from build123d import *

# Parameters (mm, degrees)
F0_W     = 10
F0_H     = 40
F0_H_2   = 20
F1_DEPTH = 120
F2_DEPTH = 30
F3_DEPTH = 100


with BuildPart() as f1:
    # F0 (on Top) → F1 (new body)
    with BuildSketch(Plane.XY):
        with Locations((5, 40)):
            Rectangle(F0_W, F0_H)
        Polygon((10, 20), (30, 20), (40, 20), (40, 40), (20, 40), (20, 60), (10, 60), align=None)
        with Locations((35, 10)):
            Rectangle(F0_W, F0_H_2)
        Polygon((0, 20), (0, 0), (30, 0), (30, 20), (10, 20), align=None)
    extrude(amount=-F1_DEPTH)

    # F0 (on Top) → F2 (cut)
    with BuildSketch(Plane.XY):
        with Locations((35, 10)):
            Rectangle(F0_W, F0_H_2)
        Polygon((10, 20), (30, 20), (40, 20), (40, 40), (20, 40), (20, 60), (10, 60), align=None)
    extrude(amount=-F2_DEPTH, mode=Mode.SUBTRACT)

    # F0 (on Top) → F3 (cut)
    with BuildSketch(Plane.XY):
        Polygon((10, 20), (30, 20), (40, 20), (40, 40), (20, 40), (20, 60), (10, 60), align=None)
    extrude(amount=-F3_DEPTH, mode=Mode.SUBTRACT)


solid = f1.part
Source: CAD feature listing. Evaluate the final solid. Frame: model axes, mm. A direction names the side the tool comes from. Give positions to 0.01 mm unless a question says otherwise; leave off trailing zeros. Write each loop counter-clockwise with the first axis right and the second up, starting at its lowest first coordinate (ties: lowest second). Pieces come first, ordered by that corner, then holes. Notation, with made-up numbers: M 75.5,7.5 L 115.5,7.5 A25 cw 115.5,29.5 Z; hole C -29.75,-27.75 d10. An arc over 180 degrees is marked long. Return JSON: item names as keys, results as strings. Group by question number.
1) Pin query (flat end, axial travel): P1, Ø10, axis at y = 53.5, z = -54.5, coming from the -X side; P2, Ø4, axis at y = 53, z = -43, coming from the +X side; P3, Ø10, axis at y = 51.5, z = -110, coming from the +X side; P4, Ø10, axis at x = 33.5, z = -110, coming from the +Y side. Return the tip coordinate at first contact, or that it passes through.
2) Cut plane A-A, the plane y = 38. Output: boundary loops of the cut face in (x, z).
3) Set-up query: faces 1 (the face through (30, 10, -15)), 2 (the face through (30, 40, -110)), 3 (the face through (21, 36, -100)). Return all of +Z, -Z, +X, -X, +Y, -Y with unobstructed straight access to the full face (end or side cutting, diameter ignored); none if empty.
4) Material intervals for line 1 along Y through (x, z) = (13, -62); line 2 along X through (y, z) = (43, -26); line 3 along Z through (x, y) = (19.5, 26), sorted ascending. Write a range as [from, to].
5) Cut plane B-B, the plane x = 12. Output: boundary loops of the cut face in (y, z), plus the area to 3 significant figures.
Recorded:
{
 "1": {"P1": "stops at x = 0", "P2": "stops at x = 10", "P3": "stops at x = 20", "P4": "stops at y = 40"},
 "2": {"outline": "M 0,-120 L 40,-120 L 40,-100 L 10,-100 L 10,0 L 0,0 Z"},
 "3": {"face 1": "+Z, +X, +Y, -Y", "face 2": "+Z, -Z, +X, +Y", "face 3": "+Z, +X, +Y"},
 "4": {"line 1": "y = [0, 20]", "line 2": "x = [0, 10]", "line 3": "z = [-120, -100]"},
 "5": {"outline": "M 0,-120 L 60,-120 L 60,-100 L 20,-100 L 20,0 L 0,0 Z", "area": "3,200 mm²"}
}
